from build123d import *

# Parameters (mm, degrees)
SKETCH1_W           = 15
SKETCH1_H           = 2.5
SKETCH1_R           = 50
BOSS_EXTRUDE1_DEPTH = 2.5


with BuildPart() as part:
    # Sketch1 → Boss-Extrude1 (new body)
    with BuildSketch(Plane.XY):
        Polygon((473.97260274, -110.342465753), (473.97260274, -60.342465753), (476.47260274, -60.342465753), (476.47260274, -10.342465753), (473.97260274, -10.342465753), (473.97260274, 14.657534247), (448.750266435, 14.657534247), (448.750266435, 12.157534247), (398.750266435, 12.157534247), (398.750266435, 14.657534247), (348.750266435, 14.657534247), (348.750266435, 12.157534247), (298.750266435, 12.157534247), (298.750266435, 14.657534247), (248.750266435, 14.657534247), (248.750266435, 12.157534247), (198.750266435, 12.157534247), (198.750266435, 14.657534247), (148.750266435, 14.657534247), (148.750266435, 12.157534247), (98.750266435, 12.157534247), (98.750266435, 14.657534247), (48.750266435, 14.657534247), (48.750266435, 12.157534247), (-1.02739726, 12.157534247), (-1.02739726, 14.657534247), (-26.02739726, 14.657534247), (-26.02739726, -10.342465753), (-28.52739726, -10.342465753), (-28.52739726, -60.342465753), (-26.02739726, -60.342465753), (-26.02739726, -110.342465753), (-28.52739726, -110.342465753), (-28.52739726, -160.342465753), (-26.02739726, -160.342465753), (-26.02739726, -210.342465753), (-28.52739726, -210.342465753), (-28.52739726, -260.342465753), (-26.02739726, -260.342465753), (-26.02739726, -310.342465753), (-28.52739726, -310.342465753), (-28.52739726, -360.342465753), (-26.02739726, -360.342465753), (-26.02739726, -410.342465753), (-28.52739726, -410.342465753), (-28.52739726, -460.342465753), (-26.02739726, -460.342465753), (-26.02739726, -487.842465753), (473.97260274, -487.842465753), (473.97260274, -460.342465753), (476.47260274, -460.342465753), (476.47260274, -410.342465753), (473.97260274, -410.342465753), (473.97260274, -360.342465753), (476.47260274, -360.342465753), (476.47260274, -310.342465753), (473.97260274, -310.342465753), (473.97260274, -260.342465753), (476.47260274, -260.342465753), (476.47260274, -210.342465753), (473.97260274, -210.342465753), (473.97260274, -160.342465753), (476.47260274, -160.342465753), (476.47260274, -110.342465753), align=None)
        with Locations((-8.52739726, -385.592465753)):
            Rectangle(SKETCH1_W, SKETCH1_H, mode=Mode.SUBTRACT)
        with Locations((73.97260274, -237.842465753)):
            Circle(SKETCH1_R, mode=Mode.SUBTRACT)
        with Locations((456.47260274, -385.592465753)):
            Rectangle(SKETCH1_W, SKETCH1_H, mode=Mode.SUBTRACT)
        with Locations((373.97260274, -237.842465753)):
            Circle(SKETCH1_R, mode=Mode.SUBTRACT)
        with Locations((-8.52739726, -85.592465753)):
            Rectangle(SKETCH1_W, SKETCH1_H, mode=Mode.SUBTRACT)
        with Locations((456.47260274, -85.592465753)):
            Rectangle(SKETCH1_W, SKETCH1_H, mode=Mode.SUBTRACT)
    extrude(amount=BOSS_EXTRUDE1_DEPTH)


solid = part.part
Source: CAD feature listing. Evaluate the final solid. Frame: model axes, mm. Coordinates: 2 decimals unless noted, no trailing zeros. Loops run counter-clockwise (first coordinate to the right, second up) from the corner with the lowest first, then second, coordinate; pieces in that order, holes last. Notation, with made-up numbers: (18.5, -23.75) - (37.5, -23.75) arc R18 ccw to (37.5, 3.25) - close; hole circle Ø3 at (87, 80.25). An arc over 180 degrees is marked (long way). One line per item, written item: value. Start each with the question number.
1. Section A-A (x = 356.5). Return the cut outline in (y, z).
2. Section B-B (x = 72.5). Return the cut outline in (y, z).
3. Contact query for flat-ended pins moving along their axis: P1, Ø1.2, axis at y = 13.5, z = 1, coming from the +X side; P2, Ø1, axis at x = 166, y = -125, coming from the -Z side; P3, Ø0.8, axis at x = -28, z = 1, coming from the +Y side; P4, Ø0.8, axis at x = 475, z = 1.5, coming from the -Y side. Output: stop coordinate, or through.
4. Ray query, L1, parallel to Y at x = -4.5, z = 0.1; L2, parallel to X at y = -251, z = 0.85; L3, parallel to X at y = -203, z = 0.8. Return the intervals inside material, ascending.
5. Mould query, pull axis Y, two halves, no side actions, for faces 1 (the cylindrical face through (121.664, -222.824, 1.232)), 2 (the flat face through (220, -233, 0)). Classes: pulls with the +Y half, pulls with the -Y half, needs draft (parallel to the pull), parting line crosses it, or undercut.
6. Section C-C (z = 1.3). State how many separate pieces and enclosed holes the cut face has, and give its area (3 significant figures).
Verdict:
1. outline: (-487.84, 0) - (-284.69, 0) - (-284.69, 2.5) - (-487.84, 2.5) - close; (-190.99, 0) - (14.66, 0) - (14.66, 2.5) - (-190.99, 2.5) - close
2. outline: (-487.84, 0) - (-287.82, 0) - (-287.82, 2.5) - (-487.84, 2.5) - close; (-187.86, 0) - (14.66, 0) - (14.66, 2.5) - (-187.86, 2.5) - close
3. P1: stops at x = 473.97
3. P2: stops at z = 0
3. P3: stops at y = -10.34
3. P4: stops at y = -460.34
4. L1: y = -487.84 to -386.84, -384.34 to -86.84, -84.34 to 14.66
4. L2: x = -28.53 to 25.73, 122.21 to 325.73, 422.21 to 476.47
4. L3: x = -26.03 to 38.11, 109.83 to 338.11, 409.83 to 473.97
5. face 1: undercut
5. face 2: needs draft
6. separate pieces: 1
6. enclosed holes: 6
6. area: 236,000 mm2
